Part model, mm, in its own coordinate system. A direction names the side the tool comes from. Give positions to 0.01 mm unless a question says otherwise; leave off trailing zeros. Loops run counter-clockwise (first coordinate to the right, second up) from the corner with the lowest first, then second, coordinate; pieces in that order, holes last. Notation, with made-up numbers: M 68,-16.75 L 80,-16.75 A34 cw 80,16.25 Z; hole C 80,-2 d2. An arc over 180 degrees is marked long. Put each result on its own line as item: value. Start each with the question number.
Solid Edge part; units mm, degrees
sketch "Sketch1" plane through (0, 0, 0) normal (0, -1, 0) x (1, 0, 0)
  circle A0 centre (0, 0) radius 5
extrude "Protrusion1" add sketch "Sketch1" along normal mid plane 115
sketch "Sketch2" plane through (0, 0, 0) normal (0, -1, 0) x (1, 0, 0)
  circle A0 centre (0, 0) radius 3
extrude "ExtrudedProtrusion_2" add sketch "Sketch2" along normal mid plane 143
sketch "Sketch3" plane through (0, -71.5, 0) normal (0, -1, 0) x (1, 0, 0)
  circle A0 centre (0, 0) radius 1.5
extrude "ExtrudedCutout_1" cut sketch "Sketch3" against normal blind 15
sketch "Sketch4" plane through (0, 71.5, 0) normal (0, 1, 0) x (0, 0, -1)
  circle A0 centre (0, 0) radius 1.5
extrude "ExtrudedCutout_2" cut sketch "Sketch4" against normal blind 15
properties material "Aluminum, 5050"
1) Pin check, flat tips, straight feed: pin 1 Ø2.5 at (x, z) = (0, 0) entering from +Y; pin 2 Ø4 at (y, z) = (3.5, -0.5) entering from -X; pin 3 Ø2.5 at (x, z) = (0, 0) entering from -Y; pin 4 Ø1 at (y, z) = (26.5, -2) entering from +X. Stop position of each tip, or through.
2) Band-saw the part on A-A on z = 0. Give the cut face in (x, y), then the cut area to 3 significant figures.
3) Which spindle directions (+Z, -Z, +X, -X, +Y, -Y) get a long thin tool onto all of the face, cutting with end or side? Do faces 1 (the flat face through (-1.3, -71.5, -1.3)), 2 (the cylindrical face through (-0.07, 64.1, 1.5)), 3 (the flat face through (0, -56.5, 0)). Say none if no direction does.
4) Mould opens along X. For faces 4 (the cylindrical face through (-1.5, -64.1, 0.07)), 5 (the flat face through (0.1, -57.5, -3.3)), 6 (the cylindrical face through (-3, -64, 0)) say: +X half, -X half, draft (parallel to the pull), parting line (faces both ways), or undercut.
5) Wall check: L1, parallel to Z at x = 0, y = -64.5; L2, parallel to Y at x = 2.75, z = 2; L3, parallel to Z at x = 4, y = -20.5. Give the ranges that are in metal, low to high.
6) Band-saw the part on C-C on y = -18.5. Give the cut face in (x, z), then the cut area to 3 significant figures.
7) Band-saw the part on B-B on x = 0. Give the cut face in (y, z).
Evaluation:
1. pin 1: y = 56.5
1. pin 2: x = -5
1. pin 3: y = -56.5
1. pin 4: x = 4.77
2. outline: M -5,-57.5 L -3,-57.5 L -3,-71.5 L -1.5,-71.5 L -1.5,-56.5 L 1.5,-56.5 L 1.5,-71.5 L 3,-71.5 L 3,-57.5 L 5,-57.5 L 5,57.5 L 3,57.5 L 3,71.5 L 1.5,71.5 L 1.5,56.5 L -1.5,56.5 L -1.5,71.5 L -3,71.5 L -3,57.5 L -5,57.5 Z
2. area: 1,230 mm2
3. face 1: +Z, -Z, +X, -X, -Y
3. face 2: +Y
3. face 3: -Y
4. face 4: undercut
4. face 5: draft
4. face 6: parting line
5. L1: -3 to -1.5, 1.5 to 3
5. L2: -57.5 to 57.5
5. L3: -3 to 3
6. outline: C 0,0 d10
6. area: 78.5 mm2
7. outline: M -71.5,-3 L -57.5,-3 L -57.5,-5 L 57.5,-5 L 57.5,-3 L 71.5,-3 L 71.5,-1.5 L 56.5,-1.5 L 56.5,1.5 L 71.5,1.5 L 71.5,3 L 57.5,3 L 57.5,5 L -57.5,5 L -57.5,3 L -71.5,3 L -71.5,1.5 L -56.5,1.5 L -56.5,-1.5 L -71.5,-1.5 Z
